from build123d import *

# Parameters (mm, degrees)
F0_R     = 25
F1_DEPTH = 7
F5_R     = 1.5
F6_DEPTH = 7.001
F8_DEPTH = 7.001


with BuildPart() as f1:
    # F0 (on Front) → F1 (new body)
    with BuildSketch(Plane.XZ):
        Circle(F0_R)
    extrude(amount=F1_DEPTH)

    # F2 (on Right) → F4 (revolve, cut)
    with BuildSketch(Plane.YZ):
        with BuildLine():
            Line((-1, 25), (-6, 25))
            ThreePointArc((-6, 25), (-3.5, 23), (-1, 25))
        make_face()
    revolve(axis=Axis((0, -8.172696, 0), (0, -1, 0)), mode=Mode.SUBTRACT)

    # F5 (on face) → F6 (cut, through all)
    with BuildSketch(Plane(origin=(0, 0, 0), x_dir=(-1, 0, 0), z_dir=(0, 1, 0))):
        Circle(F5_R)
    extrude(amount=-F6_DEPTH, mode=Mode.SUBTRACT)

    # F7 (on face) → F8 (cut, through all)
    with BuildSketch(Plane.XZ.offset(7)):
        with BuildLine():
            Line((-21, 2), (-2, 2))
            Line((-2, 2), (-2, 21))
            ThreePointArc((-2, 21), (-15.435029, 15.435029), (-21, 2))
        make_face()
        with BuildLine():
            Line((2, 21), (2, 2))
            Line((2, 2), (21, 2))
            ThreePointArc((21, 2), (15.435029, 15.435029), (2, 21))
        make_face()
        with BuildLine():
            Line((2, -2), (2, -21))
            ThreePointArc((2, -21), (15.435029, -15.435029), (21, -2))
            Line((21, -2), (2, -2))
        make_face()
        with BuildLine():
            ThreePointArc((-21, -2), (-15.435029, -15.435029), (-2, -21))
            Line((-2, -21), (-2, -2))
            Line((-2, -2), (-21, -2))
        make_face()
    extrude(amount=-F8_DEPTH, mode=Mode.SUBTRACT)


solid = f1.part
Part model, mm, in its own coordinate system. A direction names the side the tool comes from. Coordinates: 2 decimals unless noted, no trailing zeros. Loops run counter-clockwise (first coordinate to the right, second up) from the corner with the lowest first, then second, coordinate; pieces in that order, holes last. Notation, with made-up numbers: M -32,-27.75 L -11,-27.75 A26 cw -11,-0.75 Z; hole C 76,27 d7. An arc over 180 degrees is marked long. Use a Markdown table: item, result. Add a question column.
Q1. Mould opens along X. For faces 3 (the flat face through (0, 0, -5)), 4 (the flat face through (12, -4, -2)), 5 (the cylindrical face through (23.09, -6.49, -9.58)) say: +X half, -X half, draft (parallel to the pull), parting line (faces both ways), or undercut.
Q2. Probe L1, parallel to Z at x = -14, y = -2.25; L2, parallel to Z at x = -8.5, y = -5.5; L3, parallel to X at y = -4.25, z = -8. List the from-to ranges inside material, lowest first.
Q3. Pin check, flat tips, straight feed: P1, Ø3, axis at y = -4, z = 11, coming from the -X side; P2, Ø3.5, axis at x = 7.5, y = -3.5, coming from the -Z side; P3, Ø2, axis at x = 7, y = -3, coming from the +Z side. Stop position of each tip, or through.
Q4. Cut at C-C (z = 0). Write the cut outline in (x, y) (1 decimal).
Q5. Which spindle directions (+Z, -Z, +X, -X, +Y, -Y) get a long thin tool onto all of the face, cutting with end or side? Do faces 1 (the flat face through (-11, -4, -2)), 2 (the flat face through (0, -7, -5)). Say none if no direction does.
Q6. Cut at B-B (y = -3.5). Write the cut outline in (x, z).
Q7. Cut at A-A (x = 0). Write the cut outline in (y, z) (1 decimal).
Q8. Cut at D-D (z = -19). Give the number of separate pieces and of enclosed holes in the cut face, and give its area (3 significant figures).
Worked out:
| question | item | result |
|---|---|---|
| 1 | face 3 | draft |
| 1 | face 4 | undercut |
| 1 | face 5 | parting line |
| 2 | L1 | z = -18.66 to -16.73, -2 to 2, 16.73 to 18.66 |
| 2 | L2 | z = -22.4 to -19.85, -2 to 2, 19.85 to 22.4 |
| 2 | L3 | x = -21.68 to -20.03, -2 to 2, 20.03 to 21.68 |
| 3 | P1 | stops at x = -21.43 |
| 3 | P2 | stops at z = -22.57 |
| 3 | P3 | stops at z = 22.48 |
| 4 | outline | M -25,-7 L -1.5,-7 L -1.5,0 L -25,0 L -25,-1 A2.6 cw -25,-6 Z; M 1.5,-7 L 25,-7 L 25,-6 A2.6 cw 25,-1 L 25,0 L 1.5,0 Z |
| 5 | face 1 | +Y, -Y |
| 5 | face 2 | +Z, -Z, +X, -X, -Y |
| 6 | outline | C 0,0 d46; hole M -21,-2 A19 ccw -2,-21 L -2,-2 Z; hole M -21,2 L -2,2 L -2,21 A19 ccw Z; hole C 0,0 d3; hole M 2,-21 A19 ccw 21,-2 L 2,-2 Z; hole M 2,2 L 21,2 A19 ccw 2,21 Z |
| 7 | outline | M -7,-25 L -6,-25 A2.6 cw -1,-25 L 0,-25 L 0,-1.5 L -7,-1.5 Z; M -7,1.5 L 0,1.5 L 0,25 L -1,25 A2.6 cw -6,25 L -7,25 Z |
| 8 | separate pieces | 3 |
| 8 | enclosed holes | 0 |
| 8 | area | 84.5 mm2 |
